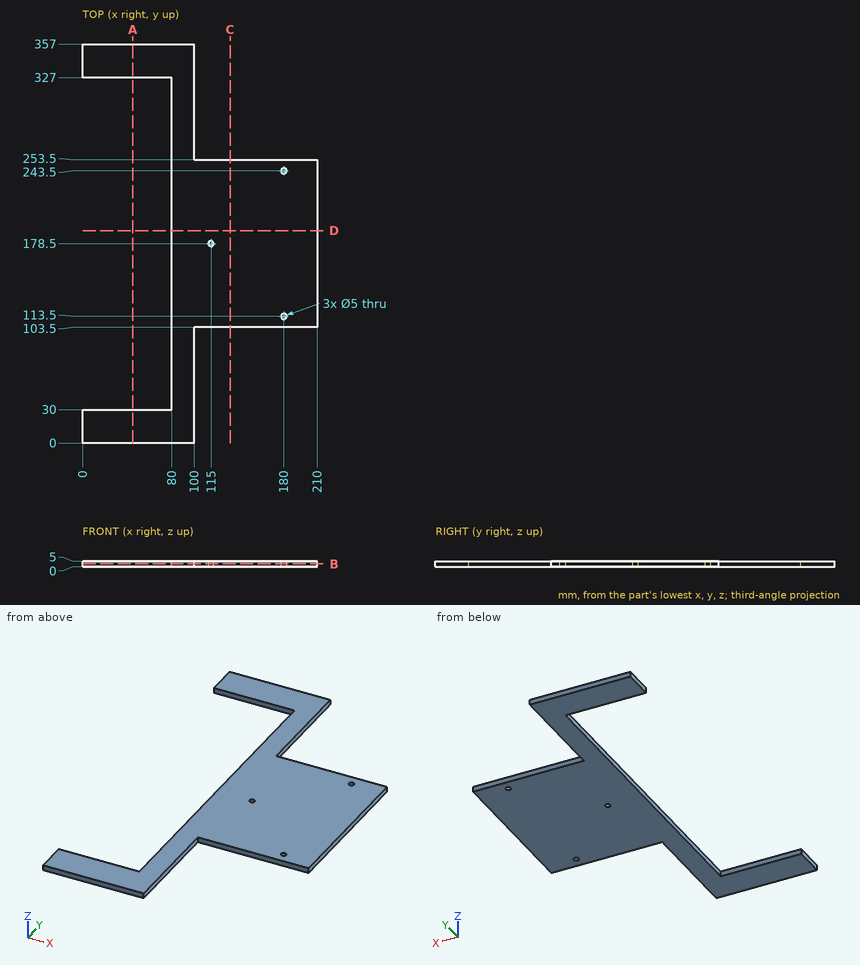
Geometry: see drawing. Coordinates: mm, zero at the bounding-box minimum. Give positions to 0.01 mm unless a question says otherwise; leave off trailing zeros. Loops run counter-clockwise (first coordinate to the right, second up) from the corner with the lowest first, then second, coordinate; pieces in that order, holes last. Notation, with made-up numbers: M 86.5,88.5 L 145.5,88.5 A18 cw 145.5,98.5 Z; hole C 17.5,-30 d9. An arc over 180 degrees is marked long. Use one line per item in the form item = value.
1. Line query: L1, parallel to Y at x = 180, z = 1.3; L2, parallel to X at y = 113.5, z = 1.1; L3, parallel to Y at x = 53, z = 1.95. Output: solid intervals per line, ascending.
Numbers:
L1 = 103.5 to 111, 116 to 241, 246 to 253.5
L2 = 80 to 177.5, 182.5 to 210
L3 = 0 to 30, 327 to 357
2. Section query B-B, the plane z = 2.7. Return the cut outline in (x, y).
Numbers:
outline = M 0,0 L 100,0 L 100,103.5 L 210,103.5 L 210,253.5 L 100,253.5 L 100,357 L 0,357 L 0,327 L 80,327 L 80,30 L 0,30 Z; hole C 115,178.5 d5; hole C 180,113.5 d5; hole C 180,243.5 d5
3. Section query D-D, the plane y = 190. Return the cut outline in (x, z), and give its area (3 significant figures).
Numbers:
outline = M 80,0 L 210,0 L 210,5 L 80,5 Z
area = 650 mm²
4. Section query C-C, the plane x = 132. Return the cut outline in (y, z).
Numbers:
outline = M 103.5,0 L 253.5,0 L 253.5,5 L 103.5,5 Z
5. First-contact query: pin 1 (3 mm diameter, centred on x = 180, y = 243.5, fed in from +Z); pin 2 (3 mm diameter, centred on x = 135, z = 4, fed in from -Y). Flat tips, straight axial feed; report the tip coordinate or a pass-through.
Numbers:
pin_1 = through
pin_2 = 103.5
6. Section query A-A, the plane x = 45. Return the cut outline in (y, z).
Numbers:
outline = M 0,0 L 30,0 L 30,5 L 0,5 Z; M 327,0 L 357,0 L 357,5 L 327,5 Z
